Source: CAD feature listing. Evaluate the final solid. Frame: model axes, mm. A direction names the side the tool comes from. Give positions to 0.01 mm unless a question says otherwise; leave off trailing zeros. Answer as a JSON object with one key per item and string values. Group by question number.
from build123d import *

# Parameters (mm, degrees)
SKETCH1_R                                           = 125
BOSS_EXTRUDE1_DEPTH                                 = 50
SKETCH2_R                                           = 127
SKETCH2_R_2                                         = 119
PAKNING_DEPTH                                       = 10
SKETCH3_R                                           = 125
SKETCH3_R_2                                         = 112
PAKNINGSRING_DEPTH                                  = 3
SKETCH5_R                                           = 5
VARMELEMENT_DEPTH                                   = 45
VARMEELEMENT_PATTERN_COUNT                          = 4
SKETCH6_R                                           = 1.5
CUT_EXTRUDE5_DEPTH                                  = 47
SKETCH7_R                                           = 135
SKETCH7_R_2                                         = 110
CUT_EXTRUDE6_DEPTH                                  = 30
CHAMFER1_SIZE                                       = 7
CHAMFER2_SIZE                                       = 0.5
M12_TAPPED_HOLE1_D                                  = 10.2
M12_TAPPED_HOLE1_DEPTH                              = 20.25
M12_TAPPED_HOLE1_TIP                                = 3.064389157
SKETCH13_R                                          = 8
CUT_EXTRUDE8_DEPTH                                  = 20
CBORE_FOR_M8_HEX_SOCKET_HEAD_CAP_SCREW1_D           = 9
CBORE_FOR_M8_HEX_SOCKET_HEAD_CAP_SCREW1_CBORE_D     = 15
CBORE_FOR_M8_HEX_SOCKET_HEAD_CAP_SCREW1_CBORE_DEPTH = 10.6
CIRPATTERN1_COUNT                                   = 4
CHAMFER3_SIZE                                       = 4
CIRPATTERN2_COUNT                                   = 8
SKETCH18_R                                          = 2.5
CUT_EXTRUDE9_DEPTH                                  = 10
CIRPATTERN3_COUNT                                   = 2


with BuildPart() as part:
    # Sketch1 → Boss-Extrude1 (new body)
    with BuildSketch(Plane(origin=(0, 0, 0), x_dir=(1, 0, 0), z_dir=(0, 1, 0))):
        Circle(SKETCH1_R)
    extrude(amount=BOSS_EXTRUDE1_DEPTH)

    # Sketch2 → Pakning (cut)
    with BuildSketch(Plane(origin=(0, 50, 0), x_dir=(1, 0, 0), z_dir=(0, 1, 0))):
        Circle(SKETCH2_R)
        Circle(SKETCH2_R_2, mode=Mode.SUBTRACT)
    extrude(amount=-PAKNING_DEPTH, mode=Mode.SUBTRACT)

    # Sketch3 → PakningsRing (cut)
    with BuildSketch(Plane(origin=(0, 50, 0), x_dir=(1, 0, 0), z_dir=(0, 1, 0))):
        Circle(SKETCH3_R)
        Circle(SKETCH3_R_2, mode=Mode.SUBTRACT)
    extrude(amount=-PAKNINGSRING_DEPTH, mode=Mode.SUBTRACT)

    # Sketch5 → Varmelement (cut)
    with BuildSketch(Plane(origin=(0, 0, 0), x_dir=(-1, 0, 0), z_dir=(0, -1, 0))):
        with Locations((-42.426406871, 42.426406871)):
            Circle(SKETCH5_R)
    varmelement = extrude(amount=-VARMELEMENT_DEPTH, mode=Mode.SUBTRACT)

    # Varmeelement_pattern: Varmelement ×4 about axis
    varmeelement_pattern_axis = Axis((0, 0, 0), (0, 1, 0))
    for i in range(1, VARMEELEMENT_PATTERN_COUNT):
        add(varmelement.rotate(varmeelement_pattern_axis, i * 360 / VARMEELEMENT_PATTERN_COUNT), mode=Mode.SUBTRACT)

    # Sketch6 → Cut-Extrude5 (cut)
    with BuildSketch(Plane.XZ):
        with Locations((14.142135624, 14.142135624)):
            Circle(SKETCH6_R)
    extrude(amount=-CUT_EXTRUDE5_DEPTH, mode=Mode.SUBTRACT)

    # Sketch7 → Cut-Extrude6 (cut)
    with BuildSketch(Plane.XZ):
        Circle(SKETCH7_R)
        Circle(SKETCH7_R_2, mode=Mode.SUBTRACT)
    extrude(amount=-CUT_EXTRUDE6_DEPTH, mode=Mode.SUBTRACT)

    # Chamfer1
    chamfer1_edges = [part.edges().sort_by_distance(p)[0] for p in [
        (-125, 30, 0),
    ]]
    chamfer(chamfer1_edges, length=CHAMFER1_SIZE)

    # Chamfer2
    chamfer2_edges = [part.edges().sort_by_distance(p)[0] for p in [
        (-119, 47, 0),
        (-112, 50, 0),
    ]]
    chamfer(chamfer2_edges, length=CHAMFER2_SIZE)

    # M12 Tapped Hole1
    with Locations(Plane(origin=(0, 0, 0), x_dir=(-1, 0, 0), z_dir=(0, -1, 0))):
        with Locations((0, 0)):
            Hole(M12_TAPPED_HOLE1_D / 2, depth=M12_TAPPED_HOLE1_DEPTH)
            with Locations((0, 0, -(M12_TAPPED_HOLE1_DEPTH + M12_TAPPED_HOLE1_TIP / 2))):  # 118° drill point
                Cone(0, M12_TAPPED_HOLE1_D / 2, M12_TAPPED_HOLE1_TIP, mode=Mode.SUBTRACT)

    # Sketch13 → Cut-Extrude8 (cut)
    with BuildSketch(Plane(origin=(0, 0, 0), x_dir=(-1, 0, 0), z_dir=(0, -1, 0))):
        with Locations((0, 95)):
            Circle(SKETCH13_R)
    cut_extrude8 = extrude(amount=-CUT_EXTRUDE8_DEPTH, mode=Mode.SUBTRACT)

    # CBORE for M8 Hex Socket Head Cap Screw1 (through all)
    with Locations(Plane(origin=(0, 50, 0), x_dir=(1, 0, 0), z_dir=(0, 1, 0))):
        with Locations((0, 95)):
            cbore_for_m8_hex_socket_head_cap_screw1 = CounterBoreHole(CBORE_FOR_M8_HEX_SOCKET_HEAD_CAP_SCREW1_D / 2, CBORE_FOR_M8_HEX_SOCKET_HEAD_CAP_SCREW1_CBORE_D / 2, CBORE_FOR_M8_HEX_SOCKET_HEAD_CAP_SCREW1_CBORE_DEPTH)

    # CirPattern1: Cut-Extrude8, CBORE for M8 Hex Socket Head Cap Screw1 ×4 about axis
    cirpattern1_axis = Axis((0, 0, 0), (0, 1, 0))
    for i in range(1, CIRPATTERN1_COUNT):
        add(cut_extrude8.rotate(cirpattern1_axis, i * 360 / CIRPATTERN1_COUNT), mode=Mode.SUBTRACT)
        add(cbore_for_m8_hex_socket_head_cap_screw1.rotate(cirpattern1_axis, i * 360 / CIRPATTERN1_COUNT), mode=Mode.SUBTRACT)

    # Chamfer3
    chamfer3_edges = [part.edges().sort_by_distance(p)[0] for p in [
        (-110, 0, 0),
    ]]
    chamfer(chamfer3_edges, length=CHAMFER3_SIZE)

    # Sketch17 → M3 Tapped Hole1 (revolve, cut)
    with BuildSketch(Plane(origin=(0, 47, -115.5), x_dir=(0, 0, 1), z_dir=(1, 0, 0))):
        Polygon((0, 0), (0, 8.251075774), (1.25, 7.5), (1.25, 0), align=None)
    m3_tapped_hole1 = revolve(axis=Axis((0, 53.35, -115.5), (0, -1, 0)), mode=Mode.SUBTRACT)

    # CirPattern2: M3 Tapped Hole1 ×8 about axis, 2 skipped
    cirpattern2_axis = Axis((0, 0, 0), (0, 1, 0))
    add([m3_tapped_hole1.rotate(cirpattern2_axis, i * 360 / CIRPATTERN2_COUNT) for i in range(1, CIRPATTERN2_COUNT) if i not in (3, 7)], mode=Mode.SUBTRACT)

    # Sketch18 → Cut-Extrude9 (cut)
    with BuildSketch(Plane(origin=(0, 47, 0), x_dir=(1, 0, 0), z_dir=(0, 1, 0))):
        with Locations((81.670833227, 81.670833227)):
            Circle(SKETCH18_R)
    cut_extrude9 = extrude(amount=-CUT_EXTRUDE9_DEPTH, mode=Mode.SUBTRACT)

    # CirPattern3: Cut-Extrude9 ×2 about axis
    cirpattern3_axis = Axis((0, 0, 0), (0, 1, 0))
    for i in range(1, CIRPATTERN3_COUNT):
        add(cut_extrude9.rotate(cirpattern3_axis, i * 360 / CIRPATTERN3_COUNT), mode=Mode.SUBTRACT)


solid = part.part
(1) Section query A-A on y = 34. State how many separate pieces and enclosed holes the cut face has, plus the area to 3 significant figures.
(2) Material intervals for line 1 (Z direction, x = 0, y = 14); line 2 (Z direction, x = -6, y = 9); line 3 (Z direction, x = 42, y = 7.5), sorted ascending. Write a range as from..to.
(3) First-contact query: pin 1 (12 mm diameter, centred on x = -96.5, y = 40, fed in from +Z) (3 decimals); pin 2 (2 mm diameter, centred on x = 81.67, z = 81.67, fed in from +Y); pin 3 (3 mm diameter, centred on x = 115.5, z = 0, fed in from +Y); pin 4 (8 mm diameter, centred on x = -95, z = 0, fed in from +Y). Flat tips, straight axial feed; report the tip coordinate or a pass-through.
(4) Access query for faces 1 (the face through (-3.69, 9.86, -87.9)), 2 (the face through (95, 39.4, 5)). Directions: +Z, -Z, +X, -X, +Y, -Y. A direction counts if a zero-diameter tool reaches every point of the face in a straight line with its end or side. Return the directions, or none.
(5) Mould query, pull axis Z, two halves, no side actions, for faces 3 (the face through (-84.272, 0.194, -64.618)), 4 (the face through (42, 45, -42)), 5 (the face through (105, 47, 43)). Classes: pulls with the +Z half, pulls with the -Z half, needs draft (parallel to the pull), parting line crosses it, or undercut.
Result:
{
 "1": {"separate pieces": "1", "enclosed holes": "9", "area": "46,200 mm²"},
 "2": {"line 1": "-110..-103, -87..-5.1, 5.1..87, 103..110", "line 2": "-109.84..-100.29, -89.71..89.71, 100.29..109.84", "line 3": "-101.67..-47.41, -37.44..37.44, 47.41..101.67"},
 "3": {"pin 1": "z = 86.225", "pin 2": "y = 39.35", "pin 3": "y = 47", "pin 4": "through"},
 "4": {"face 1": "-Y", "face 2": "+Y"},
 "5": {"face 3": "parting line crosses it", "face 4": "undercut", "face 5": "needs draft"}
}
